The model under review builds one solid part; all positions refer to its coordinate system, in mm. A direction names the side the tool comes from. Round coordinates to 2 decimals unless told otherwise and drop trailing zeros. Loops run counter-clockwise (first coordinate to the right, second up) from the corner with the lowest first, then second, coordinate; pieces in that order, holes last. Notation, with made-up numbers: (71, 17.25) -> (127, 17.25) arc R30 ccw to (127, 54.25) -> close; hole circle Ø11 at (-34, -22). An arc over 180 degrees is marked (long way). Return JSON: item names as keys, results as strings. Group by question number.
```python
from build123d import *

# Parameters (mm, degrees)
F1_DEPTH = 12
F2_R     = 2
F3_DEPTH = 132.551


with BuildPart() as f1:
    # F0 (on Top) → F1 (new body)
    with BuildSketch(Plane.XY):
        with BuildLine():
            ThreePointArc((-4.25, 0), (0, 4.25), (4.25, 0))
            Line((4.25, 0), (4.25, -20.9875))
            ThreePointArc((4.25, -20.9875), (6.007359, -25.230141), (10.25, -26.9875))
            Line((10.25, -26.9875), (120.55, -26.9875))
            ThreePointArc((120.55, -26.9875), (124.792641, -25.230141), (126.55, -20.9875))
            Line((126.55, -20.9875), (126.55, 22.225))
            Line((126.55, 22.225), (145.75, 22.225))
            ThreePointArc((145.75, 22.225), (150, 26.475), (154.25, 22.225))
            Line((154.25, 22.225), (156, 22.225))
            ThreePointArc((156, 22.225), (154.242641, 26.467641), (150, 28.225))
            Line((150, 28.225), (128.55, 28.225))
            ThreePointArc((128.55, 28.225), (124.307359, 26.467641), (122.55, 22.225))
            Line((122.55, 22.225), (122.55, -22.9875))
            Line((122.55, -22.9875), (8.25, -22.9875))
            Line((8.25, -22.9875), (8.25, 0))
            ThreePointArc((8.25, 0), (6.492641, 4.242641), (2.25, 6))
            Line((2.25, 6), (0, 6))
            ThreePointArc((0, 6), (-4.242641, 4.242641), (-6, 0))
            Line((-6, 0), (-4.25, 0))
        make_face()
    extrude(amount=F1_DEPTH)

    # F2 (on face) → F3 (cut, through all)
    with BuildSketch(Plane.YZ.offset(126.55)):
        with Locations((-8.2875, 6)):
            Circle(F2_R)
    extrude(amount=-F3_DEPTH, mode=Mode.SUBTRACT)


solid = f1.part
```
1. We need section C-C, the plane x = 67.5. Write out the cut boundary in (y, z), then the cut area to 3 significant figures.
2. Draft analysis for pull direction Z (two halves, no side actions). For faces 6 (the face through (122.55, 0, 6)), 7 (the face through (93, -24, 0)), 8 (the face through (6.278, -9.762, 7.352)), state which applies: pulls with the +Z half, pulls with the -Z half, needs draft (parallel to the pull), parting line crosses it, or undercut.
3. For P1, Ø5, axis at y = -8.29, z = 6, coming from the +X side; P2, Ø0.9, axis at x = -5, z = 8, coming from the -Y side; P3, Ø1.8, axis at x = 0.5, z = 4.5, coming from the +Y side; P4, Ø6, axis at y = -2, z = 7, coming from the -X side, all flat-tipped, find the tip position at first contact; note any pin that passes through.
4. Tool access review of faces 1 (the face through (154.29, 26.42, 5.92)), 2 (the face through (139, 28.225, 6)), 3 (the face through (136, 22.225, 6)), 4 (the face through (6.539, 4.196, 5.916)), 5 (the face through (4.25, -10.3, 4.6)): name each direction out of +Z, -Z, +X, -X, +Y, -Y from which nothing blocks a thin tool from reaching the whole face with its end or side.
5. Wall thickness on line 1 (X direction, y = -20.5, z = 5.5); line 2 (X direction, y = 2, z = 3.75): over which ranges is each line inside the solid? List them lowest first.
6. We need section B-B, the plane y = -17. Write out the cut boundary in (x, z).
7. We need section A-A, the plane z = 6. Give the number of separate pieces and of enclosed holes in the cut face, then the cut area to 3 significant figures.
Check sheet entries:
{
 "1": {"outline": "(-26.99, 0) -> (-22.99, 0) -> (-22.99, 12) -> (-26.99, 12) -> close", "area": "48.0 mm²"},
 "2": {"face 6": "needs draft", "face 7": "pulls with the -Z half", "face 8": "undercut"},
 "3": {"P1": "stops at x = 126.55", "P2": "stops at y = 0", "P3": "stops at y = 6", "P4": "stops at x = -6"},
 "4": {"face 1": "+Z, -Z, +X, +Y", "face 2": "+Z, -Z, +X, -X, +Y", "face 3": "+Z, -Z, +X, -Y", "face 4": "+Z, -Z, +Y", "face 5": "+Z, -Z, -X, -Y"},
 "5": {"line 1": "x = 4.25 to 8.25, 122.55 to 126.55", "line 2": "x = -5.66 to -3.75, 3.75 to 7.91, 122.55 to 126.55"},
 "6": {"outline": "(4.25, 0) -> (8.25, 0) -> (8.25, 12) -> (4.25, 12) -> close; (122.55, 0) -> (126.55, 0) -> (126.55, 12) -> (122.55, 12) -> close"},
 "7": {"separate pieces": "3", "enclosed holes": "0", "area": "913 mm²"}
}
